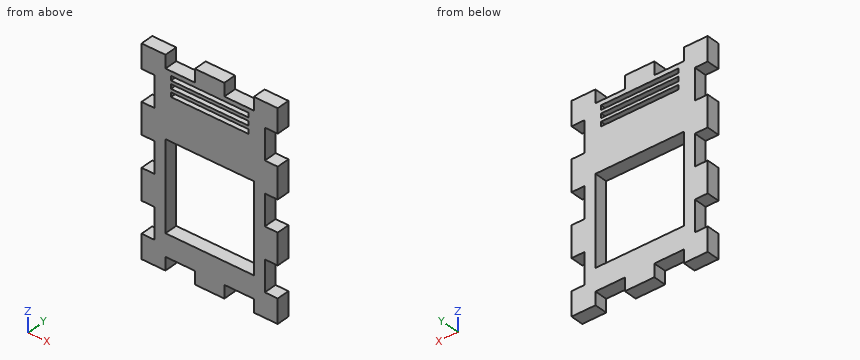
from build123d import *

# Parameters (mm, degrees)
F0_W     = 40
F0_H     = 40
F0_W_2   = 35
F0_H_2   = 2
F1_DEPTH = 5.842


with BuildPart() as f1:
    # F0 (on Front) → F1 (new body)
    with BuildSketch(Plane.XZ):
        Polygon((-20, -45.842), (-20, -40), (-6.666667, -40), (-6.666667, -45.842), (6.666667, -45.842), (6.666667, -40), (20, -40), (20, -45.842), (30.842, -45.842), (30.842, -35), (25, -35), (25, -21), (30.842, -21), (30.842, -7), (25, -7), (25, 7), (30.842, 7), (30.842, 21), (25, 21), (25, 35), (30.842, 35), (30.842, 45.842), (20, 45.842), (20, 40), (6.666667, 40), (6.666667, 45.842), (-6.666667, 45.842), (-6.666667, 40), (-20, 40), (-20, 45.842), (-30.842, 45.842), (-30.842, 35), (-25, 35), (-25, 21), (-30.842, 21), (-30.842, 7), (-25, 7), (-25, -7), (-30.842, -7), (-30.842, -21), (-25, -21), (-25, -35), (-30.842, -35), (-30.842, -45.842), align=None)
        with Locations((0, -10)):
            Rectangle(F0_W, F0_H, mode=Mode.SUBTRACT)
        with Locations((0, 30)):
            Rectangle(F0_W_2, F0_H_2, mode=Mode.SUBTRACT)
        with Locations((0, 33.5)):
            Rectangle(F0_W_2, F0_H_2, mode=Mode.SUBTRACT)
        with Locations((0, 37)):
            Rectangle(F0_W_2, F0_H_2, mode=Mode.SUBTRACT)
    extrude(amount=F1_DEPTH)


solid = f1.part
The model under review builds one solid part; all positions refer to its coordinate system, in mm. Coordinates: 2 decimals unless noted, no trailing zeros. Loops run counter-clockwise (first coordinate to the right, second up) from the corner with the lowest first, then second, coordinate; pieces in that order, holes last. Notation, with made-up numbers: M 83,-0.75 L 137,-0.75 A25 cw 137,33.25 Z; hole C 57,-4 d11. An arc over 180 degrees is marked long. Put each result on its own line as item: value. Start each with the question number.
Q1. Add section D-D (x = 5.5). Write out the cut boundary in (y, z), and give its area (3 significant figures).
Q2. Clearance check with flat-ended pins moving along their axes: pin 1 (2 mm diameter, centred on y = -1, z = -34.5, fed in from +X); pin 2 (1.8 mm diameter, centred on y = -3.5, z = -26, fed in from +X); pin 3 (3 mm diameter, centred on x = 11.5, y = -4, fed in from -Z); pin 4 (1 mm diameter, centred on y = -2.5, z = 1.5, fed in from -X). State where each tip first meets the part, or that it passes through.
Q3. Add section B-B (x = -27). Write out the cut boundary in (y, z), and give its area (3 significant figures).
Q4. Add section C-C (x = -15.5). Write out the cut boundary in (y, z), and give its area (3 significant figures).
Q5. Wall thickness on line 1 (Z direction, x = 27.5, y = -4.9); line 2 (Z direction, x = -1.5, y = -2.95); line 3 (Z direction, x = 9, y = -2.25): over which ranges is each line inside the solid? List them lowest first.
Q6. Add section A-A (z = 8). Write out the cut boundary in (x, y).
Answers:
1. outline: M -5.84,-45.84 L 0,-45.84 L 0,-30 L -5.84,-30 Z; M -5.84,10 L 0,10 L 0,29 L -5.84,29 Z; M -5.84,31 L 0,31 L 0,32.5 L -5.84,32.5 Z; M -5.84,34.5 L 0,34.5 L 0,36 L -5.84,36 Z; M -5.84,38 L 0,38 L 0,45.84 L -5.84,45.84 Z
1. area: 267 mm^2
2. pin 1: stops at x = 30.84
2. pin 2: stops at x = 25
2. pin 3: stops at z = -40
2. pin 4: stops at x = -25
3. outline: M -5.84,-45.84 L 0,-45.84 L 0,-35 L -5.84,-35 Z; M -5.84,-21 L 0,-21 L 0,-7 L -5.84,-7 Z; M -5.84,7 L 0,7 L 0,21 L -5.84,21 Z; M -5.84,35 L 0,35 L 0,45.84 L -5.84,45.84 Z
3. area: 290 mm^2
4. outline: M -5.84,-40 L 0,-40 L 0,-30 L -5.84,-30 Z; M -5.84,10 L 0,10 L 0,29 L -5.84,29 Z; M -5.84,31 L 0,31 L 0,32.5 L -5.84,32.5 Z; M -5.84,34.5 L 0,34.5 L 0,36 L -5.84,36 Z; M -5.84,38 L 0,38 L 0,40 L -5.84,40 Z
4. area: 199 mm^2
5. line 1: z = -45.84 to -35, -21 to -7, 7 to 21, 35 to 45.84
5. line 2: z = -45.84 to -30, 10 to 29, 31 to 32.5, 34.5 to 36, 38 to 45.84
5. line 3: z = -40 to -30, 10 to 29, 31 to 32.5, 34.5 to 36, 38 to 40
6. outline: M -30.84,-5.84 L -20,-5.84 L -20,0 L -30.84,0 Z; M 20,-5.84 L 30.84,-5.84 L 30.84,0 L 20,0 Z
